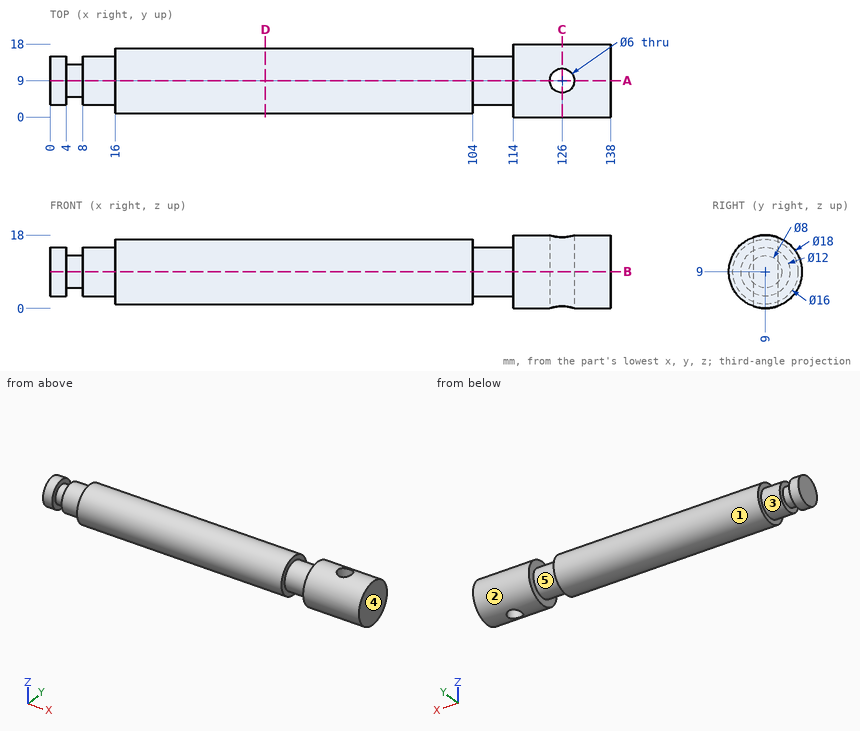
Job drawing, mm, ordinate dimensions from the low corner. One solid piece. A direction names the side the tool comes from. Give positions to 0.01 mm unless a question says otherwise; leave off trailing zeros. Write each loop counter-clockwise with the first axis right and the second up, starting at its lowest first coordinate (ties: lowest second). Pieces come first, ordered by that corner, then holes. Notation, with made-up numbers: (11, 8) - (41, 8) arc R24 ccw to (41, 42) - close; hole circle Ø5 at (-2, -32). An arc over 180 degrees is marked (long way). Use one line per item in the form item = value. Start each with the question number.
1. Drop flat-ended pins along their axis: pin 1 Ø10 at (x, z) = (96, 13.5) entering from +Y; pin 2 Ø10 at (x, z) = (40.5, 15.5) entering from +Y; pin 3 Ø3 at (x, z) = (15.5, 9.5) entering from -Y. Give the stop position or say it passes through.
2. Band-saw the part on B-B on z = 9. Write the cut outline in (x, y).
3. Probe line 1 (X direction, y = 2.5, z = 12); line 2 (X direction, y = 9, z = 4.5); line 3 (X direction, y = 9.25, z = 10.5). List the from-to ranges inside material, lowest first. Write a range as [from, to].
4. Band-saw the part on A-A on y = 9. Write the cut outline in (x, z).
5. Band-saw the part on C-C on x = 126. Write the cut outline in (y, z).
6. Two-plate mould, pull along X, no slides. Class the marked faces 3, 4 and 5: released by +X, released by -X, zero draft, split by the parting line, or undercut.
7. Band-saw the part on D-D on x = 53. Write the cut outline in (y, z), plus the area to 3 significant figures.
8. 3-axis set-ups, long thin cutter, end or side, ignore diameter. For the marked faces 1 and 2: which of +Z, -Z, +X, -X, +Y, -Y reach the whole face in a straight line?
Conclusion:
q1.pin_1 = 17
q1.pin_2 = 16.86
q1.pin_3 = 1
q2.outline = (0, 3) - (4, 3) - (4, 5) - (8, 5) - (8, 3) - (16, 3) - (16, 1) - (104, 1) - (104, 3) - (114, 3) - (114, 0) - (138, 0) - (138, 18) - (114, 18) - (114, 15) - (104, 15) - (104, 17) - (16, 17) - (16, 15) - (8, 15) - (8, 13) - (4, 13) - (4, 15) - (0, 15) - close; hole circle Ø6 at (126, 9)
q3.line_1 = [16, 104], [114, 138]
q3.line_2 = [0, 4], [8, 123], [129, 138]
q3.line_3 = [0, 123.01], [128.99, 138]
q4.outline = (0, 3) - (4, 3) - (4, 5) - (8, 5) - (8, 3) - (16, 3) - (16, 1) - (104, 1) - (104, 3) - (114, 3) - (114, 0) - (123, 0) - (123, 18) - (114, 18) - (114, 15) - (104, 15) - (104, 17) - (16, 17) - (16, 15) - (8, 15) - (8, 13) - (4, 13) - (4, 15) - (0, 15) - close; (129, 0) - (138, 0) - (138, 18) - (129, 18) - close
q5.outline = (6, 0.51) - (6, 17.49) arc R9 ccw to start; (12, 0.51) arc R9 ccw to (12, 17.49) - close
q6.face_3 = zero draft
q6.face_4 = released by +X
q6.face_5 = undercut
q7.outline = circle Ø16 at (9, 9)
q7.area = 201 mm²
q8.face_1 = -X
q8.face_2 = +X, -X
